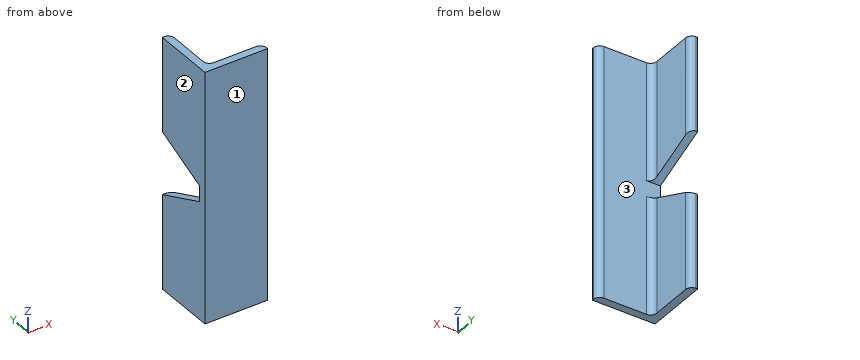
from build123d import *

# Parameters (mm, degrees)
BOSS_EXTRUDE1_DEPTH = 50.8
CUT_EXTRUDE1_DEPTH  = 59.198711326


with BuildPart() as part:
    # Sketch1 → Boss-Extrude1 (new, symmetric)
    with BuildSketch(Plane.XY):
        with BuildLine():
            Line((-12.7, 12.7), (-12.7, -12.7))
            Line((-12.7, -12.7), (12.7, -12.7))
            Line((12.7, -12.7), (12.7, -12.065))
            ThreePointArc((12.7, -12.065), (11.956051224, -10.268948776), (10.16, -9.525))
            Line((10.16, -9.525), (-6.985, -9.525))
            ThreePointArc((-6.985, -9.525), (-8.781051224, -8.781051224), (-9.525, -6.985))
            Line((-9.525, -6.985), (-9.525, 10.16))
            ThreePointArc((-9.525, 10.16), (-10.268948776, 11.956051224), (-12.065, 12.7))
            Line((-12.065, 12.7), (-12.7, 12.7))
        make_face()
    extrude(amount=BOSS_EXTRUDE1_DEPTH, both=True)

    # Sketch3 → Cut-Extrude1 (cut, through all)
    with BuildSketch(Plane.ZY.offset(12.7)):
        Polygon((-12.7, 12.7), (-3.175, -9.525), (3.175, -9.525), (12.7, 12.7), align=None)
    extrude(amount=-CUT_EXTRUDE1_DEPTH, mode=Mode.SUBTRACT)


solid = part.part
Verification items for the finished model (mm, model axes). Face numbers are marked on the shaded views. Give positions to 0.01 mm unless a question says otherwise; leave off trailing zeros. Write each loop counter-clockwise with the first axis right and the second up, starting at its lowest first coordinate (ties: lowest second). Pieces come first, ordered by that corner, then holes. Notation, with made-up numbers: M 43.25,1 L 71.25,1 A11 ccw 71.25,8 Z; hole C 11,88.25 d2. An arc over 180 degrees is marked long. Write item = value, one per line.
(1) Go/stop test with flat-tipped pins: pin 1 Ø6 at (y, z) = (8, -8) entering from +X (3 decimals); pin 2 Ø13.5 at (y, z) = (-1, 37) entering from +X; pin 3 Ø2 at (y, z) = (-3.5, -4.5) entering from -X; pin 4 Ø1.5 at (x, z) = (2.5, 37) entering from +Y (3 decimals). Record where each tip stops, or that it passes through.
Found:
pin_1 = -9.525
pin_2 = -9.41
pin_3 = through
pin_4 = -9.525
(2) Sectioned sample at B-B (z = -17). Record the cut outline in (x, y) (3 decimals).
Found:
outline = M -12.7,-12.7 L 12.7,-12.7 L 12.7,-12.065 A2.54 ccw 10.16,-9.525 L -6.985,-9.525 A2.54 cw -9.525,-6.985 L -9.525,10.16 A2.54 ccw -12.065,12.7 L -12.7,12.7 Z
(3) Material ranges on line 1 (X direction, y = -5.5, z = 39) (3 decimals); line 2 (X direction, y = -11, z = 2.5), recorded low to high.
Found:
line_1 = -12.7 to -9.525
line_2 = -12.7 to 12.47
(4) Sectioned sample at C-C (x = -10.75). Record the cut outline in (y, z) (3 decimals), then the cut area to 3 significant figures.
Found:
outline = M -12.7,-50.8 L 12.333,-50.8 L 12.333,-12.543 L -9.525,-3.175 L -9.525,3.175 L 12.333,12.543 L 12.333,50.8 L -12.7,50.8 Z
area = 2,200 mm2
(5) Draft check along Y on the marked faces 1, 2 and 3. Enter one of: released by +Y, released by -Y, zero draft, split by the parting line, or undercut.
Found:
face_1 = released by -Y
face_2 = zero draft
face_3 = released by +Y
(6) Sectioned sample at D-D (y = 7.75). Record the cut outline in (x, z) (3 decimals), then the cut area to 3 significant figures.
Found:
outline = M -12.7,-50.8 L -9.525,-50.8 L -9.525,-10.579 L -12.7,-10.579 Z; M -12.7,10.579 L -9.525,10.579 L -9.525,50.8 L -12.7,50.8 Z
area = 255 mm2
(7) Sectioned sample at A-A (y = -5). Record the cut outline in (x, z) (3 decimals).
Found:
outline = M -12.7,-50.8 L -9.525,-50.8 L -9.525,-5.114 L -12.7,-5.114 Z; M -12.7,5.114 L -9.525,5.114 L -9.525,50.8 L -12.7,50.8 Z
